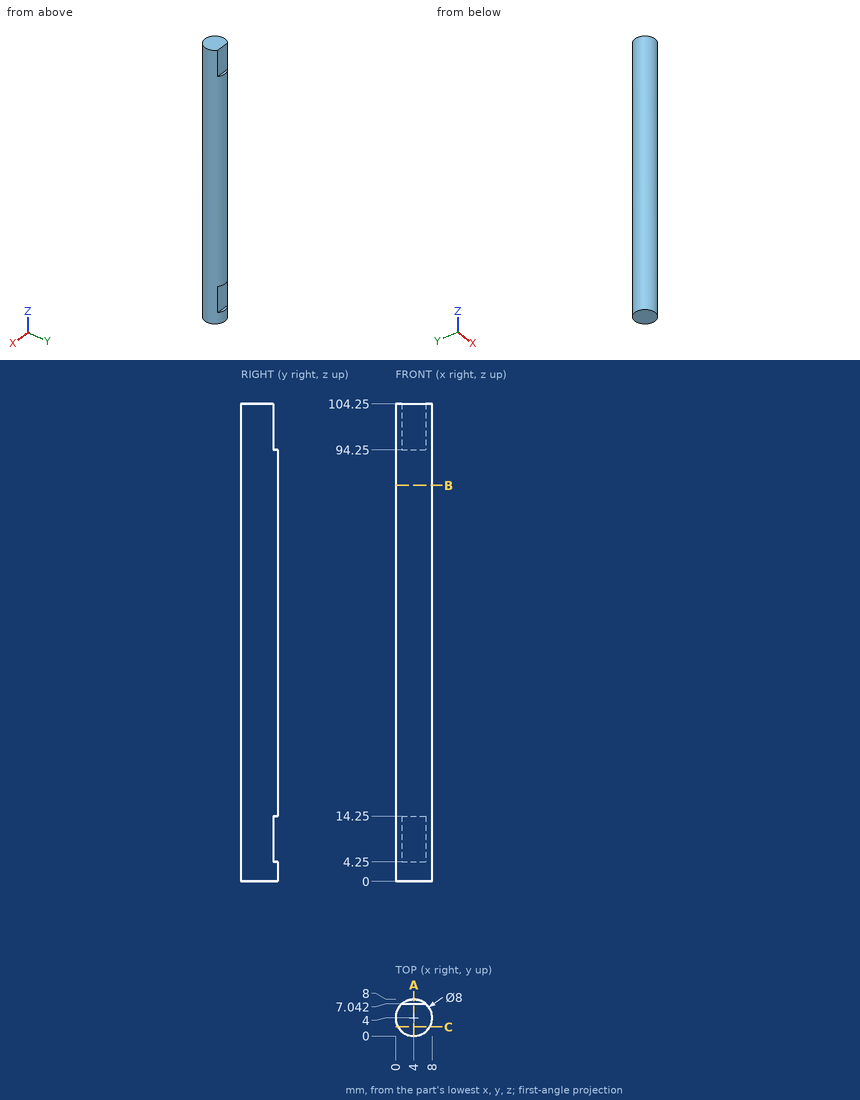
Design review of the part shown in the three views and the two pictorial views. Dimensions are in mm from the part's minimum x, y and z. Coordinates: 2 decimals unless noted, no trailing zeros. Loops run counter-clockwise (first coordinate to the right, second up) from the corner with the lowest first, then second, coordinate; pieces in that order, holes last. Notation, with made-up numbers: M 30,21 L 84,21 A21 cw 84,40 Z; hole C 34.25,-1.5 d11. An arc over 180 degrees is marked long. One line per question, with ' | ' between items.
(1) We need section C-C (y = 2). Give the boundary of the cut face in (x, z).
Filled in:
outline: M 0.54,0 L 7.46,0 L 7.46,104.25 L 0.54,104.25 Z
(2) For pin 1 Ø3 at (x, y) = (6.5, 6.5) entering from -Z; pin 2 Ø1.5 at (y, z) = (2.5, 49) entering from +X; pin 3 Ø2.5 at (x, z) = (3.5, 10) entering from +Y; pin 4 Ø1.5 at (y, z) = (5.5, 30.5) entering from -X, all flat-tipped, find the tip position at first contact; note any pin that passes through.
Filled in:
pin 1: stops at z = 0 | pin 2: stops at x = 7.93 | pin 3: stops at y = 7.04 | pin 4: stops at x = 0.07
(3) Wall thickness on probe 1 along X at (y, z) = (4.25, 73); probe 2 along Y at (x, z) = (7.25, 7); probe 3 along X at (y, z) = (5.75, 74.5): over which ranges is each line inside the solid? List them lowest first.
Filled in:
probe 1: x = 0.01 to 7.99 | probe 2: y = 1.67 to 6.33 | probe 3: x = 0.4 to 7.6
(4) We need section A-A (x = 4). Give the boundary of the cut face in (y, z), and give its area (3 significant figures).
Filled in:
outline: M 0,0 L 8,0 L 8,4.25 L 7.04,4.25 L 7.04,14.25 L 8,14.25 L 8,94.25 L 7.04,94.25 L 7.04,104.25 L 0,104.25 Z | area: 815 mm^2
(5) We need section B-B (z = 86.5). Give the boundary of the cut face in (x, y).
Filled in:
outline: C 4,4 d8
